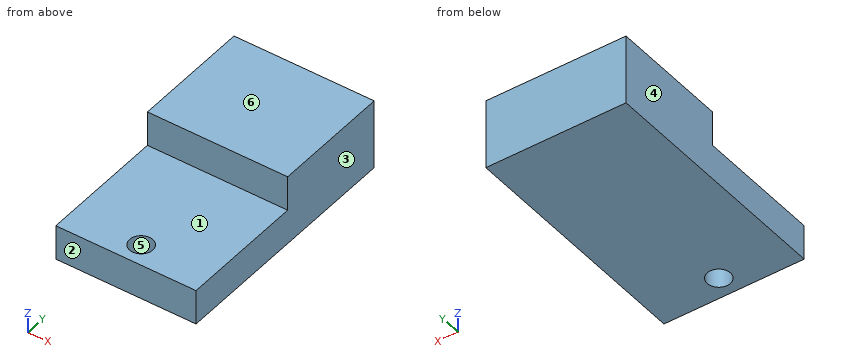
Autodesk Inventor part; units mm, degrees
ref_plane "YZ Plane" through (0, 0, 0) normal (1, 0, 0) x (0, 1, 0)
ref_plane "XZ Plane" through (0, 0, 0) normal (0, 1, 0) x (-1, 0, 0)
ref_plane "XY Plane" through (0, 0, 0) normal (0, 0, 1) x (1, 0, 0)
sketch "Skizze1" plane through (0, 0, 0) normal (0, 0, 1) x (1, 0, 0)
  line L0 (-4, 0) -> (24, 0)
  line L1 (0, -7) -> (0, 42)
  line L2 (0, 0) -> (20, 0)
  line L3 (20, 0) -> (20, 35)
  line L4 (20, 35) -> (0, 35)
  line L5 (0, 35) -> (0, 0)
  dimension "d0" = 35
  dimension "d1" = 20
extrude "Extrusion1" add sketch "Skizze1" along normal blind 10
sketch "Skizze2" plane through (0, 0, 10) normal (0, 0, 1) x (1, 0, 0)
  line L0 (0, 0) -> (20, 0)
  line L1 (20, 0) -> (20, 35)
  point P0 (10, 3)
  dimension "d4" = 10
  dimension "d5" = 3
hole "Bohrung1" at (10, 3, 10) direction (0, 0, -1) diameter 3.3 end through all
sketch "Skizze3" plane through (20, 0, 0) normal (1, 0, 0) x (0, 0, -1)
  line L0 (-10, 0) -> (-5, 0)
  line L1 (-5, 0) -> (-5, 18)
  line L2 (-5, 18) -> (-10, 18)
  line L3 (-10, 18) -> (-10, 0)
  dimension "d13" = 5
  dimension "d14" = 18
extrude "Extrusion2" cut sketch "Skizze3" against normal through all
properties part number "Platine" material "Edelstahl"
Check sheet for the modelled part. Datum: model origin and axes. Units: mm. Face numbers are marked on the shaded views. A direction names the side the tool comes from. Round coordinates to 2 decimals unless told otherwise and drop trailing zeros. Order: outer loops, then holes, each group sorted by start corner. A loop starts at its lowest first (then second) coordinate and runs counter-clockwise, first axis right, second up.
1) Go/stop test with flat-tipped pins: pin 1 Ø4 at (x, z) = (12, 8) entering from -Y; pin 2 Ø3 at (y, z) = (25.5, 6.5) entering from -X; pin 3 Ø2 at (x, y) = (10, 3) entering from -Z. Record where each tip stops, or that it passes through.
2) Scan lines: line 1 (Y direction, x = 10, z = 3.1); line 2 (X direction, y = 3, z = 2); line 3 (Y direction, x = 8, z = 9). Record each from-to range of solid material in increasing order.
3) Section check B-B (y = 3). Record the boundary of the cut face in (x, z), and give its area (3 significant figures).
4) Section check C-C (x = 15). Record the boundary of the cut face in (y, z).
5) Tool access check on the marked faces 1 and 2. Record the directions out of +Z, -Z, +X, -X, +Y, -Y that give a thin tool (end or side, any length) a straight path to the whole face; none if there is none.
6) Mould release check, pull along X, two halves, no side actions. Record for the marked faces 3, 4, 5 and 6: +X half, -X half, draft (parallel to the pull), parting line (faces both ways), or undercut.
7) Section check A-A (x = 10). Record the boundary of the cut face in (y, z), and give its area (4 significant figures).
8) Section check D-D (z = 7). Record the boundary of the cut face in (x, y).
Result:
1. pin 1: stops at y = 18
1. pin 2: stops at x = 0
1. pin 3: passes through
2. line 1: y = 0 to 1.35, 4.65 to 35
2. line 2: x = 0 to 8.35, 11.65 to 20
2. line 3: y = 18 to 35
3. outline: (0, 0) - (8.35, 0) - (8.35, 5) - (0, 5) - close; (11.65, 0) - (20, 0) - (20, 5) - (11.65, 5) - close
3. area: 83.5 mm2
4. outline: (0, 0) - (35, 0) - (35, 10) - (18, 10) - (18, 5) - (0, 5) - close
5. face 1: +Z, +X, -X, -Y
5. face 2: +Z, -Z, +X, -X, -Y
6. face 3: +X half
6. face 4: -X half
6. face 5: undercut
6. face 6: draft
7. outline: (0, 0) - (1.35, 0) - (1.35, 5) - (0, 5) - close; (4.65, 0) - (35, 0) - (35, 10) - (18, 10) - (18, 5) - (4.65, 5) - close
7. area: 243.5 mm2
8. outline: (0, 18) - (20, 18) - (20, 35) - (0, 35) - close
